Build history of the part. All positions in model axes, mm. A direction names the side the tool comes from. Give positions to 0.01 mm unless a question says otherwise; leave off trailing zeros. Loops run counter-clockwise (first coordinate to the right, second up) from the corner with the lowest first, then second, coordinate; pieces in that order, holes last. Notation, with made-up numbers: M -5.5,39 L 11.5,39 A25 cw 11.5,73 Z; hole C -23.5,2 d8. An arc over 180 degrees is marked long. Answer as a JSON object with one key per item and string values. Group by question number.
1. Drill centre lines: line 1 along X through (y, z) = (-4.5, 0) (3 decimals); line 2 along X through (y, z) = (-4.75, 25). Where is each one in solid material? Low to high. Write a range as [from, to].
2. Slice it at D-D (z = -26). List the corners of the cut face in (x, y), then the cut area to 3 significant figures.
3. Mould opens along Z. For faces 5 (the face through (-54, -3, -24.13)), 6 (the face through (-57.963, -3, 17)), 7 (the face through (-51, -3, 20.447)) say: released by +Z, released by -Z, zero draft, split by the parting line, or undercut.
4. Slice it at A-A (z = 22.5). List the corners of the cut face in (x, y).
5. Slice it at B-B (x = 0). List the corners of the cut face in (y, z) (3 decimals).
6. Drop flat-ended pins along their axis: pin 1 Ø1.9 at (x, y) = (-40, -2.5) entering from +Z; pin 2 Ø12 at (x, z) = (-36, 29) entering from +Y; pin 3 Ø3 at (x, y) = (-54, -2.5) entering from -Z; pin 4 Ø1.9 at (y, z) = (-2, -28) entering from -X. Give the stop position or say it passes through.
7. 3-axis set-ups, long thin cutter, end or side, ignore diameter. For faces 1 (the face through (-46.203, -3, -22)), 2 (the face through (-48, -3, -17.78)), 3 (the face through (-48, -3, -9.931)), 4 (the face through (-49.86, -3, 22)): which of +Z, -Z, +X, -X, +Y, -Y reach the whole face in a straight line?
from build123d import *

# Parameters (mm, degrees)
SKETCH1_R           = 6.985
BOSS_EXTRUDE1_DEPTH = 6.35


with BuildPart() as part:
    # Sketch1 → Boss-Extrude1 (new body)
    with BuildSketch(Plane(origin=(0, 0, 0), x_dir=(1, 0, 0), z_dir=(0, 1, 0))):
        Polygon((-38.1, -38.1), (38.1, -38.1), (38.1, 38.1), (-38.1, 38.1), (-38.1, 24.13), (-46.2026, 24.13), (-46.2026, 20.447), (-44.0944, 20.447), (-44.0944, 17.78), (-51.9684, 17.78), (-51.9684, 20.447), (-49.8602, 20.447), (-49.8602, 24.13), (-57.9628, 24.13), (-57.9628, 9.9314), (-38.1, 9.9314), (-38.1, -9.9314), (-57.9628, -9.9314), (-57.9628, -24.13), (-49.8602, -24.13), (-49.8602, -20.447), (-51.9684, -20.447), (-51.9684, -17.78), (-44.0944, -17.78), (-44.0944, -20.447), (-46.2026, -20.447), (-46.2026, -24.13), (-38.1, -24.13), align=None)
        Circle(SKETCH1_R, mode=Mode.SUBTRACT)
    extrude(amount=-BOSS_EXTRUDE1_DEPTH)


solid = part.part
Established:
{
 "1": {"line 1": "x = [-38.1, -6.985], [6.985, 38.1]", "line 2": "x = [-38.1, 38.1]"},
 "2": {"outline": "M -38.1,-6.35 L 38.1,-6.35 L 38.1,0 L -38.1,0 Z", "area": "484 mm^2"},
 "3": {"face 5": "released by -Z", "face 6": "zero draft", "face 7": "undercut"},
 "4": {"outline": "M -57.96,-6.35 L -49.86,-6.35 L -49.86,0 L -57.96,0 Z; M -46.2,-6.35 L 38.1,-6.35 L 38.1,0 L -46.2,0 Z"},
 "5": {"outline": "M -6.35,-38.1 L 0,-38.1 L 0,-6.985 L -6.35,-6.985 Z; M -6.35,6.985 L 0,6.985 L 0,38.1 L -6.35,38.1 Z"},
 "6": {"pin 1": "stops at z = 24.13", "pin 2": "stops at y = 0", "pin 3": "stops at z = -24.13", "pin 4": "stops at x = -38.1"},
 "7": {"face 1": "-Z, +Y, -Y", "face 2": "+Y, -Y", "face 3": "-X, +Y, -Y", "face 4": "+Z, +Y, -Y"}
}
